Can you work these out from the model? Positions are in its coordinate system, mm. Coordinates: 2 decimals unless noted, no trailing zeros. Write each loop counter-clockwise with the first axis right and the second up, starting at its lowest first coordinate (ties: lowest second). Pieces come first, ordered by that corner, then holes. Notation, with made-up numbers: (34.25, 27.5) - (48.25, 27.5) arc R32 cw to (48.25, 56.5) - close; hole circle Ø1 at (-3, -40). An arc over 180 degrees is marked (long way). Use one line per item in the form item = value. Start each with the question number.
(1) If we section it at A-A on y = 0: Please give me the cut outline in (x, z), then the cut area to 3 significant figures.
(2) Thinking about a two-plate mould opening in Y: for faces 1 (the face through (-1, -57.15, 1)), 2 (the face through (-38.1, -1, 1)), 3 (the face through (-5.86, 11.267, -0.533)), which applies, pulls with the +Y half, pulls with the -Y half, needs draft (parallel to the pull), parting line crosses it, or undercut?
(3) If I drill on probe 1 along Y at (x, z) = (0, -7.5); probe 2 along Y at (x, z) = (-2.5, -34); probe 3 along X at (y, z) = (-8.5, -11.5), over which ranges is the centre line in solid material (lowest first)? Write a range as from..to.
(4) If we section it at B-B on x = 0: Please give me the cut outline in (y, z).
(5) If we section it at C-C on z = -16: Please give me the cut outline in (x, y).
```python
from build123d import *

# Parameters (mm, degrees)
SKETCH1_W           = 76.2
SKETCH1_H           = 114.3
SKETCH1_R           = 12.7
BOSS_EXTRUDE1_DEPTH = 38.1


with BuildPart() as part:
    # Sketch1 → Boss-Extrude1 (new, symmetric)
    with BuildSketch(Plane.XY):
        Rectangle(SKETCH1_W, SKETCH1_H)
        with Locations(Location((0, 0, 0), (0, 0, 180))):
            Circle(SKETCH1_R, mode=Mode.SUBTRACT)
    extrude(amount=BOSS_EXTRUDE1_DEPTH, both=True)


solid = part.part
```
Reported:
q1.outline = (-38.1, -38.1) - (-12.7, -38.1) - (-12.7, 38.1) - (-38.1, 38.1) - close; (12.7, -38.1) - (38.1, -38.1) - (38.1, 38.1) - (12.7, 38.1) - close
q1.area = 3,870 mm2
q2.face_1 = pulls with the -Y half
q2.face_2 = needs draft
q2.face_3 = undercut
q3.probe_1 = -57.15..-12.7, 12.7..57.15
q3.probe_2 = -57.15..-12.45, 12.45..57.15
q3.probe_3 = -38.1..-9.44, 9.44..38.1
q4.outline = (-57.15, -38.1) - (-12.7, -38.1) - (-12.7, 38.1) - (-57.15, 38.1) - close; (12.7, -38.1) - (57.15, -38.1) - (57.15, 38.1) - (12.7, 38.1) - close
q5.outline = (-38.1, -57.15) - (38.1, -57.15) - (38.1, 57.15) - (-38.1, 57.15) - close; hole circle Ø25.4 at (0, 0)
